Verification items for the finished model (mm, model axes). Round coordinates to 2 decimals unless told otherwise and drop trailing zeros. Write each loop counter-clockwise with the first axis right and the second up, starting at its lowest first coordinate (ties: lowest second). Pieces come first, ordered by that corner, then holes.
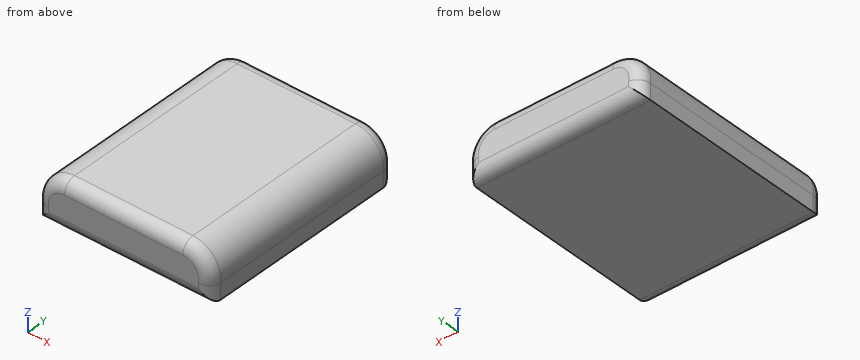
from build123d import *

# Parameters (mm, degrees)
F0_W     = 30
F0_H     = 12
F1_DEPTH = 54
F2_R     = 3
F3_R     = 3


with BuildPart() as f1:
    # F0 (on Front) → F1 (new body)
    with BuildSketch(Plane.XZ):
        Rectangle(F0_W, F0_H)
        with BuildLine():
            Line((15, 6), (15, -6))
            Line((15, -6), (22, -6))
            Line((22, -6), (22, -2))
            ThreePointArc((22, -2), (20.3150729064, 3.5881887931), (15, 6))
        make_face()
        with BuildLine():
            Line((-22, -6), (-15, -6))
            Line((-15, -6), (-15, 6))
            ThreePointArc((-15, 6), (-20.3150729064, 3.5881887931), (-22, -2))
            Line((-22, -2), (-22, -6))
        make_face()
    extrude(amount=F1_DEPTH)

    # F2
    f2_edges = [f1.edges().sort_by_distance(p)[0] for p in [
        (22, -54, -4),
        (20.315073, -54, 3.588189),
        (0, -54, 6),
        (-20.315073, -54, 3.588189),
        (-22, -54, -4),
        (0, -54, -6),
    ]]
    fillet(f2_edges, radius=F2_R)

    # F3
    f3_edges = [f1.edges().sort_by_distance(p)[0] for p in [
        (22, 0, -4),
        (20.315073, 0, 3.588189),
        (0, 0, 6),
        (-20.315073, 0, 3.588189),
        (-22, 0, -4),
        (0, 0, -6),
    ]]
    fillet(f3_edges, radius=F3_R)


solid = f1.part
Q1. Material ranges on line 1 along X through (y, z) = (-10, -3.5); line 2 along X through (y, z) = (-22, -1.25); line 3 along Y through (x, z) = (13, 4), recorded low to high.
Recorded:
line 1: x = -22 to 22
line 2: x = -22.06 to 22.06
line 3: y = -53.83 to -0.17
Q2. Depth check by flat-ended pin: P1, Ø1.5, axis at y = -43.5, z = 3, coming from the +X side; P2, Ø1.2, axis at y = -27.5, z = -5, coming from the -X side; P3, Ø2, axis at y = -27, z = -4.5, coming from the +X side. Enter the tip coordinate at first touch or a pass-through.
Recorded:
P1: stops at x = 21.24
P2: stops at x = -22
P3: stops at x = 22
Q3. Sectioned sample at B-B (z = -4.25). Enter the section's corners in (x, y).
Recorded:
outline: (-22, -51) arc R3 ccw to (-20.25, -53.73) - (20.25, -53.73) arc R3 ccw to (22, -51) - (22, -3) arc R3 ccw to (20.25, -0.27) - (-20.25, -0.27) arc R3 ccw to (-22, -3) - close
Q4. Sectioned sample at A-A (y = -43). Enter the section's corners in (x, z) (1 decimal), plus the area to 3 significant figures.
Recorded:
outline: (-22, -6) - (22, -6) - (22, -2) arc R7.1 ccw to (15, 6) - (-15, 6) arc R7.1 ccw to (-22, -2) - close
area: 508 mm2
